Source: CAD feature listing. Evaluate the final solid. Frame: model axes, mm. Face numbers are marked on the shaded views. A direction names the side the tool comes from. Coordinates: 2 decimals unless noted, no trailing zeros. Order: outer loops, then holes, each group sorted by start corner. A loop starts at its lowest first (then second) coordinate and runs counter-clockwise, first axis right, second up. Notation, with made-up numbers: (12.25, 64) -> (47.25, 64) arc R8 ccw to (47.25, 77) -> close; hole circle Ø4 at (77.25, 65.25). An arc over 180 degrees is marked (long way). Write item = value, one per line. Start each with the question number.
Item 1: Section query A-A (x = 17.5). Output: boundary loops of the cut face in (y, z).
Item 2: Section query B-B (y = 0). Output: boundary loops of the cut face in (x, z), then the cut area to 3 significant figures.
Item 3: Section query C-C (z = -7.75). Output: boundary loops of the cut face in (x, y), then the cut area to 3 significant figures.
Item 4: Contact query for flat-ended pins moving along their axis: pin 1 (6 mm diameter, centred on x = -53.5, y = -15, fed in from -Z); pin 2 (4 mm diameter, centred on x = -33, y = -2, fed in from -Z); pin 3 (8 mm diameter, centred on x = -62, y = -4.5, fed in from +Z). Output: stop coordinate, or through.
Item 5: Section query D-D (x = -46.5). Output: boundary loops of the cut face in (y, z), then the cut area to 3 significant figures.
Item 6: Set-up query: the marked faces 1, 2, 3 and 4. Return all of +Z, -Z, +X, -X, +Y, -Y with unobstructed straight access to the full face (end or side cutting, diameter ignored); none if empty.
Item 7: Ray query, line 1 along Y through (x, z) = (17.5, -5.75); line 2 along Y through (x, z) = (-6, -3.5); line 3 along Y through (x, z) = (33.5, -5.75). Return the intervals inside material, ascending. Write a range as [from, to].
Item 8: Mould query, pull axis Y, two halves, no side actions, for the marked faces 5, 6, 7 and 8. Classes: released by +Y, released by -Y, zero draft, split by the parting line, or undercut.
Autodesk Inventor part; units mm, degrees
ref_plane "YZ Plane" through (0, 0, 0) normal (1, 0, 0) x (0, 1, 0)
ref_plane "XZ Plane" through (0, 0, 0) normal (0, 1, 0) x (-1, 0, 0)
ref_plane "XY Plane" through (0, 0, 0) normal (0, 0, 1) x (1, 0, 0)
sketch "Sketch1" plane through (0, 0, 0) normal (0, 0, 1) x (1, 0, 0)
  line L0 (-17.5, 13) -> (2.3013, 13)
  line L1 (2.3013, -13) -> (-17.5, -13)
  line L2 (-17.5, -13) -> (-17.5, 13)
  arc A0 (2.3013, -13) -> (2.3013, 13) centre (17.5, 0) ccw
  circle A1 centre (17.5, 0) radius 10
  point P0 (0, 0)
extrude "Extrusion1" add sketch "Sketch1" along normal mid plane 26
sketch "Sketch2" plane through (-17.5, -13, 13) normal (-1, 0, 0) x (0, 0, 1)
  line L0 (-26, 26) -> (0, 26)
  line L1 (-13, 26) -> (-1.7417, 19.5)
  line L2 (-1.7417, 19.5) -> (-1.7417, 6.5)
  line L3 (-1.7417, 6.5) -> (-13, 0)
  line L4 (-13, 0) -> (-24.2583, 6.5)
  line L5 (-24.2583, 6.5) -> (-24.2583, 19.5)
  line L6 (-24.2583, 19.5) -> (-13, 26)
  point P0 (-13, 13)
  point P1 (-13, 13)
extrude "Extrusion2" add sketch "Sketch2" along normal blind 35
sketch "Sketch3" plane through (-52.5, -13, 13) normal (-1, 0, 0) x (0, 0, 1)
  circle A0 centre (-13, 13) radius 10
extrude "Extrusion3" add sketch "Sketch3" along normal blind 30
fillet "Fillet1" radius 20 1 edges at (2.3013, 13, 0)
fillet "Fillet2" radius 20 1 edges at (2.3013, -13, 0)
chamfer "Chamfer1" distance 1 angle 45 6 edges at (-52.5, -9.75, -5.6292) (-52.5, 0, -11.2583) (-52.5, 9.75, -5.6292) (-52.5, -9.75, 5.6292) (-52.5, 0, 11.2583) (-52.5, 9.75, 5.6292)
fillet "Fillet3" radius 1 18 edges at (7.5, 0, -13) (7.5, 0, 13) (0.8108, -13.895, -13) (-11.3027, -13, -13) (0.8108, 13.895, -13) (-11.3027, 13, -13) (37.5, 0, -13) (-17.5, 0, -13) (0.8108, -13.895, 13) (37.5, 0, 13) (0.8108, 13.895, 13) (-11.3027, 13, 13) (-11.3027, -13, 13) (-17.5, 0, 13) (-17.5, -13, 6.5) (-17.5, -13, -6.5) (-17.5, 13, 6.5) (-17.5, 13, -6.5)
properties part number "Single Eye End"
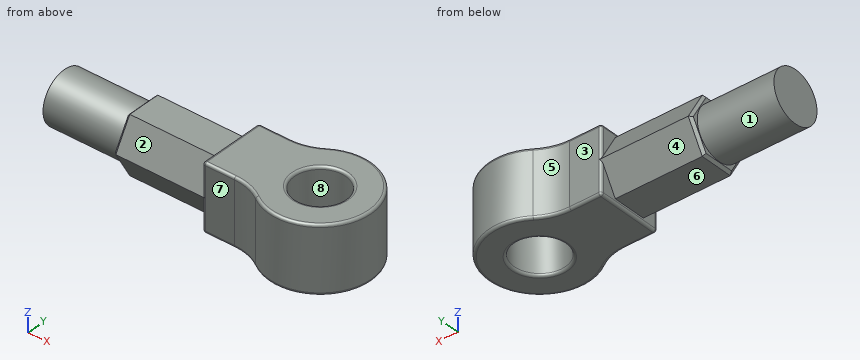
Computed:
q1.outline = (-20, -12) arc R1 ccw to (-19, -13) -> (-11, -13) arc R1 ccw to (-10, -12) -> (-10, 12) arc R1 ccw to (-11, 13) -> (-19, 13) arc R1 ccw to (-20, 12) -> close; (10, -12) arc R1 ccw to (11, -13) -> (19, -13) arc R1 ccw to (20, -12) -> (20, 12) arc R1 ccw to (19, 13) -> (11, 13) arc R1 ccw to (10, 12) -> close
q2.outline = (-82.5, -10) -> (-52.5, -10) -> (-52.5, -10.26) -> (-51.5, -11.26) -> (-17.5, -11.26) -> (-17.5, -12) arc R1 ccw to (-16.5, -13) -> (6.5, -13) arc R1 ccw to (7.5, -12) -> (7.5, 12) arc R1 ccw to (6.5, 13) -> (-16.5, 13) arc R1 ccw to (-17.5, 12) -> (-17.5, 11.26) -> (-51.5, 11.26) -> (-52.5, 10.26) -> (-52.5, 10) -> (-82.5, 10) -> close; (27.5, -12) arc R1 ccw to (28.5, -13) -> (36.5, -13) arc R1 ccw to (37.5, -12) -> (37.5, 12) arc R1 ccw to (36.5, 13) -> (28.5, 13) arc R1 ccw to (27.5, 12) -> close
q2.area = 2,300 mm^2
q3.outline = (-82.5, -6.32) -> (-52.5, -6.32) -> (-52.5, -7.37) -> (-51.5, -8.53) -> (-17.5, -8.53) -> (-17.5, -12) arc R1 ccw to (-16.5, -13) -> (-5.11, -13) arc R20 cw to (6.2, -16.5) arc R20 ccw (long way) to (6.2, 16.5) arc R20 cw to (-5.11, 13) -> (-16.5, 13) arc R1 ccw to (-17.5, 12) -> (-17.5, 8.53) -> (-51.5, 8.53) -> (-52.5, 7.37) -> (-52.5, 6.32) -> (-82.5, 6.32) -> close; hole circle Ø20 at (17.5, 0)
q3.area = 2,360 mm^2
q4.pin_1 = -0.41
q4.pin_2 = -11.26
q4.pin_3 = 9.99
q5.outline = (-13, 0) -> (-6.5, -11.26) -> (6.5, -11.26) -> (13, 0) -> (6.5, 11.26) -> (-6.5, 11.26) -> close
q5.area = 439 mm^2
q6.face_1 = -X
q6.face_2 = +Z, -X, -Y
q6.face_3 = +Z, -Z, -X, +Y
q6.face_4 = -Z, -X, +Y
q7.line_1 = [-20, -10], [10, 20]
q7.line_2 = [-13, 13]
q7.line_3 = [-12, 12]
q8.face_5 = released by +Y
q8.face_6 = zero draft
q8.face_7 = released by -Y
q8.face_8 = undercut
